```python
from build123d import *

# Parameters (mm, degrees)
SKETCH1_W           = 213.628300444
SKETCH1_H           = 8
EXTRUDE1_DEPTH      = 8
EXTRUDE2_DEPTH      = 8
LPATTERN1_COUNT     = 34
LPATTERN1_PITCH     = 6.283185307
SKETCH_1_W          = 133.268632933
SKETCH_1_H          = 8
CUT_EXTRUDE_1_DEPTH = 25
SKETCH_2_W          = 4.961443825
SKETCH_2_H          = 8
CUT_EXTRUDE_2_DEPTH = 50
SKETCH_3_W          = 80.359667511
SKETCH_3_H          = 1
CUT_EXTRUDE_3_DEPTH = 50
SKETCH_4_W          = 80.359667511
SKETCH_4_H          = 9.5
EXTRUDE_1_DEPTH     = 3.3
SKETCH_5_R          = 10.5
SKETCH_5_R_2        = 9.5
EXTRUDE_2_DEPTH     = 7
EXTRUDE_2_2_DEPTH   = 7
SKETCH_6_R          = 10.5
EXTRUDE_3_DEPTH     = 2
EXTRUDE_4_DEPTH     = 2
SKETCH_8_R          = 1.525
CUT_EXTRUDE_4_DEPTH = 2
FILLET_1_R          = 4


with BuildPart() as part:
    # Sketch1 → Extrude1 (new body)
    with BuildSketch(Plane.XY):
        with Locations((106.814150222, -4)):
            Rectangle(SKETCH1_W, SKETCH1_H)
    extrude(amount=EXTRUDE1_DEPTH)

    # Sketch2 → Extrude2 (add)
    with BuildSketch(Plane.XY.offset(8)):
        Polygon((0, 0), (1.637866054, 4.5), (3.323577771, 4.5), (4.961443825, 0), align=None)
    extrude2 = extrude(amount=-EXTRUDE2_DEPTH)

    # LPattern1: Extrude2 ×34
    with Locations(*[(i * LPATTERN1_PITCH, 0, 0) for i in range(1, LPATTERN1_COUNT)]):
        add(extrude2)

    # Sketch 1 → Cut-Extrude 1 (cut, symmetric)
    with BuildSketch(Plane(origin=(0, 0, 0), x_dir=(1, 0, 0), z_dir=(0, 1, 0))):
        with Locations((146.993983978, -4)):
            Rectangle(SKETCH_1_W, SKETCH_1_H)
    extrude(amount=CUT_EXTRUDE_1_DEPTH, both=True, mode=Mode.SUBTRACT)

    # Sketch 2 → Cut-Extrude 2 (cut)
    with BuildSketch(Plane(origin=(0, 0, 0), x_dir=(1, 0, 0), z_dir=(0, 1, 0))):
        with Locations((77.878945599, -4)):
            Rectangle(SKETCH_2_W, SKETCH_2_H)
        with Locations((2.480721912, -4)):
            Rectangle(SKETCH_2_W, SKETCH_2_H)
    extrude(amount=CUT_EXTRUDE_2_DEPTH, mode=Mode.SUBTRACT)

    # Sketch 3 → Cut-Extrude 3 (cut)
    with BuildSketch(Plane(origin=(0, 0, 0), x_dir=(-1, 0, 0), z_dir=(0, 0, -1))):
        with Locations((-40.179833756, -7.5)):
            Rectangle(SKETCH_3_W, SKETCH_3_H)
    extrude(amount=-CUT_EXTRUDE_3_DEPTH, mode=Mode.SUBTRACT)

    # Sketch 4 → Extrude 1 (add)
    with BuildSketch(Plane.XZ.offset(7)):
        with Locations((40.179833756, 12.75)):
            Rectangle(SKETCH_4_W, SKETCH_4_H)
    extrude(amount=-EXTRUDE_1_DEPTH)



with BuildPart() as body_2:
    # Sketch 5 → Extrude 2 (new body)
    with BuildSketch(Plane.XY.offset(17.5)):
        with Locations((61.879833756, -28.2)):
            Circle(SKETCH_5_R)
        with Locations((61.879833756, -28.2)):
            Circle(SKETCH_5_R_2, mode=Mode.SUBTRACT)
    extrude(amount=-EXTRUDE_2_DEPTH)


with BuildPart() as body_3:
    # Sketch 5 → Extrude 2 2 (new body)
    with BuildSketch(Plane.XY.offset(17.5)):
        with Locations((18.479833756, -28.2)):
            Circle(SKETCH_5_R)
        with Locations((18.479833756, -28.2)):
            Circle(SKETCH_5_R_2, mode=Mode.SUBTRACT)
    extrude(amount=-EXTRUDE_2_2_DEPTH)


with BuildPart() as part_1:
    add(part.part)

    add(body_2.part)  # Extrude 3 merges body 2

    add(body_3.part)  # Extrude 3 merges body 3
    # Sketch 6 → Extrude 3 (add)
    with BuildSketch(Plane.XY.offset(17.5)):
        Polygon((-3.520166244, -41.2), (83.879833756, -41.2), (83.879833756, -13.2), (80.359667511, -7), (0, -7), (-3.520166244, -13.2), align=None)
        with Locations((61.879833756, -28.2)):
            Circle(SKETCH_6_R, mode=Mode.SUBTRACT)
        with Locations((18.479833756, -28.2)):
            Circle(SKETCH_6_R, mode=Mode.SUBTRACT)
    extrude(amount=-EXTRUDE_3_DEPTH)

    # Sketch 7 → Extrude 4 (add)
    with BuildSketch(Plane.ZY.offset(3.520166244)):
        with BuildLine():
            Line((17.5, -15.2), (9.198571137, -15.2))
            ThreePointArc((9.198571137, -15.2), (7.09630212, -16.059797912), (6.199050778, -18.14635668))
            Line((6.199050778, -18.14635668), (5.950495627, -32.044568569))
            ThreePointArc((5.950495627, -32.044568569), (6.693951707, -34.11470505), (8.623569492, -35.170530414))
            ThreePointArc((8.623569492, -35.170530414), (8.836276209, -35.192623828), (9.05, -35.2))
            Line((9.05, -35.2), (17.5, -35.2))
            Line((17.5, -35.2), (17.5, -15.2))
        make_face()
    extrude_4 = extrude(amount=-EXTRUDE_4_DEPTH)

    # Mirror 1: Extrude 4 across plane
    add(extrude_4.mirror(Plane.ZY.offset(-40.179833756)))

    # Sketch 8 → Cut-Extrude 4 (cut)
    with BuildSketch(Plane.ZY.offset(3.520166244)):
        with Locations((9.3, -18.4)):
            Circle(SKETCH_8_R)
        with Locations((9.3, -32)):
            Circle(SKETCH_8_R)
    cut_extrude_4 = extrude(amount=-CUT_EXTRUDE_4_DEPTH, mode=Mode.SUBTRACT)

    # Mirror 2: Cut-Extrude 4 across plane
    add(cut_extrude_4.mirror(Plane.ZY.offset(-40.179833756)), mode=Mode.SUBTRACT)

    # Fillet 1
    fillet_1_edges = [part_1.edges().sort_by_distance(p)[0] for p in [
        (83.879833756, -41.2, 16.5),
        (-3.520166244, -41.2, 16.5),
    ]]
    fillet(fillet_1_edges, radius=FILLET_1_R)


solid = part_1.part
```
Here's how the part is built. I have some questions about the finished solid (model axes, mm). A direction names the side the tool comes from. Give positions to 0.01 mm unless a question says otherwise; leave off trailing zeros. Write each loop counter-clockwise with the first axis right and the second up, starting at its lowest first coordinate (ties: lowest second). Pieces come first, ordered by that corner, then holes.
(1) Thinking about a two-plate mould opening in X: for faces 1 (the face through (38.5, 2.2, 4.1)), 2 (the face through (80.36, -4, 7)), 3 (the face through (15, 4.5, 4)), which applies, pulls with the +X half, pulls with the -X half, needs draft (parallel to the pull), parting line crosses it, or undercut?
Output values:
face 1: undercut
face 2: pulls with the +X half
face 3: needs draft
(2) Imagine slicing it at A-A, the plane z = 12. Write out the boundary of the cut face in (x, y).
Output values:
outline: (-3.52, -35.2) - (-1.52, -35.2) - (-1.52, -15.2) - (-3.52, -15.2) - close; (0, -7) - (80.36, -7) - (80.36, -3.7) - (0, -3.7) - close; circle Ø21 at (18.48, -28.2); circle Ø21 at (61.88, -28.2); (81.88, -35.2) - (83.88, -35.2) - (83.88, -15.2) - (81.88, -15.2) - close; hole circle Ø19 at (18.48, -28.2); hole circle Ø19 at (61.88, -28.2)
(3) Imagine slicing it at B-B, the plane y = -24. Write out the boundary of the cut face in (x, z), and give its area (3 significant figures).
Output values:
outline: (-3.52, 6.09) - (-1.52, 6.09) - (-1.52, 15.5) - (8.86, 15.5) - (8.86, 10.5) - (9.96, 10.5) - (9.96, 17.5) - (-3.52, 17.5) - close; (27, 10.5) - (28.1, 10.5) - (28.1, 15.5) - (52.26, 15.5) - (52.26, 10.5) - (53.36, 10.5) - (53.36, 17.5) - (27, 17.5) - close; (70.4, 10.5) - (71.5, 10.5) - (71.5, 15.5) - (81.88, 15.5) - (81.88, 6.09) - (83.88, 6.09) - (83.88, 17.5) - (70.4, 17.5) - close
area: 166 mm2
(4) If I drill on L1, parallel to Y at x = -2.9, z = 9.3 (3 decimals); L2, parallel to X at y = -30, z = 15.75; L3, parallel to Y at x = 15, z = 13.25, over which ranges is the centre line in solid material (lowest first)?
Output values:
L1: y = -35.2 to -33.525, -30.475 to -19.925, -16.875 to -15.2
L2: x = -3.52 to 9.15, 27.81 to 52.55, 71.21 to 83.88
L3: y = -38.11 to -37.04, -19.36 to -18.29, -7 to -3.7
(5) On a 3-axis mill with a long thin cutter (end or side, diameter ignored), from which of +Z, -Z, +X, -X, +Y, -Y can I reach the whole of each face in a straight line? I mean faces 4 (the face through (-3, -15.2, 12)), 5 (the face through (51.073, 2.218, 4.056)), 6 (the face through (83, -35.2, 12)). Say none if no direction works.
Output values:
face 4: -Z, +X, -X, +Y
face 5: +Z, -Z, +Y
face 6: -Z, +X, -Y
(6) Will these pins go through, and if not, where does the flat tip stop? pin 1 (2 mm diameter, centred on y = -3.5, z = 5, fed in from +X); pin 2 (2 mm diameter, centred on x = 71.5, z = 8.5, fed in from -Y); pin 3 (1 mm diameter, centred on x = 83, z = 12, fed in from +Y).
Output values:
pin 1: stops at x = 80.36
pin 2: stops at y = -7
pin 3: stops at y = -15.2
